The model under review builds one solid part; all positions refer to its coordinate system, in mm. Face numbers are marked on the shaded views. Coordinates: 2 decimals unless noted, no trailing zeros. Write each loop counter-clockwise with the first axis right and the second up, starting at its lowest first coordinate (ties: lowest second). Pieces come first, ordered by that corner, then holes. Notation, with made-up numbers: (-35, 52) - (19, 52) arc R18 cw to (19, 75) - close; hole circle Ø4 at (-39, -7). An arc over 180 degrees is marked (long way). Put each result on its own line as item: value. Start each with the question number.
Item 1: Mouldability with a two-part tool opening along Z and no side actions: class the marked faces 1, 2 and 3 as pulls with the +Z half, pulls with the -Z half, needs draft (parallel to the pull), parting line crosses it, or undercut.
Item 2: Consider section C-C on y = 46.5. State how many separate pieces and enclosed holes the cut face has, then the cut area to 3 significant figures.
Item 3: Consider section B-B on z = 179.75. Give the boundary of the cut face in (x, y), then the cut area to 3 significant figures.
Item 4: To check wall thickness, follow L1, parallel to X at y = 69, z = 134.5; L2, parallel to X at y = 94.5, z = -184.5; L3, parallel to Y at x = -139, z = -8. State the ranges of each line that lie inside material, in increasing order. Write a range as [from, to].
Item 5: For pin 1 (3 mm diameter, centred on x = 152, y = 47.5, fed in from -Z); pin 2 (3 mm diameter, centred on x = 101.5, y = 20.5, fed in from -Z) (3 decimals); pin 3 (4 mm diameter, centred on y = 88, z = -197, fed in from +X), all flat-tipped, find the tip position at first contact; note any pin that passes through.
Item 6: Consider section A-A on x = 0. Give the boundary of the cut face in (y, z), then the cut area to 3 significant figures.
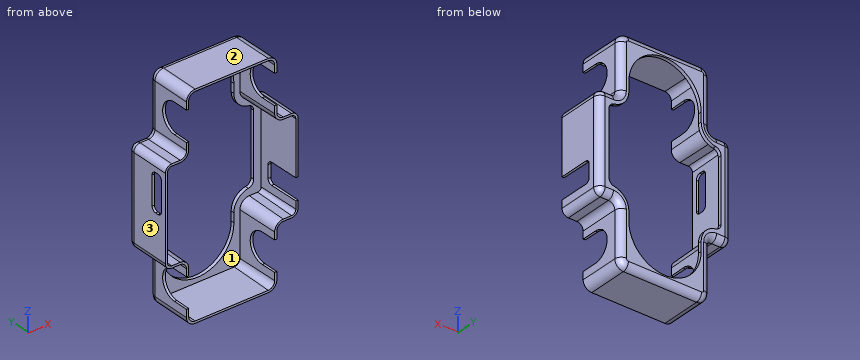
```python
from build123d import *

# Parameters (mm, degrees)
SKETCH1_W           = 310
SKETCH1_H           = 505
BOSS_EXTRUDE1_DEPTH = 108
SKETCH2_W           = 75
SKETCH2_H           = 140
CUT_EXTRUDE1_DEPTH  = 316.349409386
FILLET1_R           = 15
FILLET3_R           = 20
FILLET4_R           = 15
FILLET5_R           = 15
CUT_EXTRUDE2_DEPTH  = 379.524107555
CUT_EXTRUDE3_DEPTH  = 100
CUT_EXTRUDE3_DRAFT  = -1
SKETCH18_W          = 87
SKETCH18_H          = 27.388454903
CUT_EXTRUDE4_DEPTH  = 90
FILLET6_R           = 10
SKETCH19_W          = 50
SKETCH19_H          = 98.394535989
CUT_EXTRUDE5_DEPTH  = 90
FILLET7_R           = 10
CUT_EXTRUDE7_DEPTH  = 90
FILLET12_R          = 40
FILLET13_R          = 15


with BuildPart() as part:
    # Sketch1 → Boss-Extrude1 (new body)
    with BuildSketch(Plane(origin=(0, 0, 0), x_dir=(1, 0, 0), z_dir=(0, 1, 0))):
        Rectangle(SKETCH1_W, SKETCH1_H)
    extrude(amount=BOSS_EXTRUDE1_DEPTH)

    # Sketch2 → Cut-Extrude1 (cut, through all)
    with BuildSketch(Plane(origin=(0, 0, 0), x_dir=(-1, 0, 0), z_dir=(0, -1, 0))):
        with Locations((143, -182.5)):
            Rectangle(SKETCH2_W, SKETCH2_H)
        with Locations((-143, -182.5)):
            Rectangle(SKETCH2_W, SKETCH2_H)
        with Locations((-143, 182.5)):
            Rectangle(SKETCH2_W, SKETCH2_H)
        with Locations((143, 182.5)):
            Rectangle(SKETCH2_W, SKETCH2_H)
    extrude(amount=-CUT_EXTRUDE1_DEPTH, mode=Mode.SUBTRACT)

    # Fillet1
    fillet1_edges = [part.edges().sort_by_distance(p)[0] for p in [
        (-105.5, 54, -112.5),
        (105.5, 54, -112.5),
        (105.5, 54, 112.5),
        (-105.5, 54, 112.5),
    ]]
    fillet(fillet1_edges, radius=FILLET1_R)

    # Fillet3
    fillet3_edges = [part.edges().sort_by_distance(p)[0] for p in [
        (-105.5, 54, -252.5),
        (105.5, 54, -252.5),
        (105.5, 54, 252.5),
        (-105.5, 54, 252.5),
    ]]
    fillet(fillet3_edges, radius=FILLET3_R)

    # Fillet4
    fillet4_edges = [part.edges().sort_by_distance(p)[0] for p in [
        (105.5, 108, 180),
        (0, 108, 252.5),
        (-105.5, 108, -180),
        (0, 108, -252.5),
        (-99.642135624, 108, -246.642135624),
        (99.642135624, 108, -246.642135624),
        (-99.642135624, 108, 246.642135624),
        (99.642135624, 108, 246.642135624),
        (155, 108, 0),
        (-155, 108, 0),
        (137.75, 108, -112.5),
        (-137.75, 108, 112.5),
        (137.75, 108, 112.5),
        (-105.5, 108, 180),
        (105.5, 108, -180),
        (-137.75, 108, -112.5),
        (109.893398282, 108, 116.893398282),
        (-109.893398282, 108, 116.893398282),
        (109.893398282, 108, -116.893398282),
        (-109.893398282, 108, -116.893398282),
    ]]
    fillet(fillet4_edges, radius=FILLET4_R)

    # Fillet5
    # the kernel refuses this fillet: 15 mm, written as the material it takes off along each edge
    with BuildSketch(Plane(origin=(140, 93, -97.5), x_dir=(0, 0, -1), z_dir=(1, 0, 0))) as fillet5_piece_1_section:
        Polygon((0, 0), (FILLET5_R, 0), (FILLET5_R, FILLET5_R), (0, FILLET5_R), align=None)
    fillet5_piece_1 = extrude(amount=FILLET5_R, mode=Mode.PRIVATE)
    fillet5_piece_1 = fillet5_piece_1 - Plane(origin=(140, 93, -97.5), x_dir=(0, -0.7071067811865475, 0.7071067811865475), z_dir=(1, 0, 0)) * Sphere(FILLET5_R, mode=Mode.PRIVATE)
    add(fillet5_piece_1, mode=Mode.SUBTRACT)
    with BuildSketch(Plane(origin=(140, 93, 97.5), x_dir=(1, 0, 0), z_dir=(0, 0, 1))) as fillet5_piece_2_section:
        Polygon((0, 0), (FILLET5_R, 0), (FILLET5_R, FILLET5_R), (0, FILLET5_R), align=None)
    fillet5_piece_2 = extrude(amount=FILLET5_R, mode=Mode.PRIVATE)
    fillet5_piece_2 = fillet5_piece_2 - Plane(origin=(140, 93, 97.5), x_dir=(-0.7071067811865475, -0.7071067811865475, 0), z_dir=(0, 0, 1)) * Sphere(FILLET5_R, mode=Mode.PRIVATE)
    add(fillet5_piece_2, mode=Mode.SUBTRACT)
    with BuildSketch(Plane(origin=(-140, 93, -97.5), x_dir=(0, 0, -1), z_dir=(-1, 0, 0))) as fillet5_piece_3_section:
        Polygon((0, 0), (FILLET5_R, 0), (FILLET5_R, -FILLET5_R), (0, -FILLET5_R), align=None)
    fillet5_piece_3 = extrude(amount=FILLET5_R, mode=Mode.PRIVATE)
    fillet5_piece_3 = fillet5_piece_3 - Plane(origin=(-140, 93, -97.5), x_dir=(0, -0.7071067811865475, 0.7071067811865475), z_dir=(-1, 0, 0)) * Sphere(FILLET5_R, mode=Mode.PRIVATE)
    add(fillet5_piece_3, mode=Mode.SUBTRACT)
    with BuildSketch(Plane(origin=(-140, 93, 97.5), x_dir=(-1, 0, 0), z_dir=(0, 0, 1))) as fillet5_piece_4_section:
        Polygon((0, 0), (FILLET5_R, 0), (FILLET5_R, -FILLET5_R), (0, -FILLET5_R), align=None)
    fillet5_piece_4 = extrude(amount=FILLET5_R, mode=Mode.PRIVATE)
    fillet5_piece_4 = fillet5_piece_4 - Plane(origin=(-140, 93, 97.5), x_dir=(0.7071067811865475, -0.7071067811865475, 0), z_dir=(0, 0, 1)) * Sphere(FILLET5_R, mode=Mode.PRIVATE)
    add(fillet5_piece_4, mode=Mode.SUBTRACT)
    with BuildSketch(Plane(origin=(155, 93, 112.5), x_dir=(-1, 0, 0), z_dir=(0, -1, 0)), Plane(origin=(155, 93, -112.5), x_dir=(0, 0, 1), z_dir=(0, -1, 0))) as fillet5_piece_5:
        with BuildLine():
            CenterArc((FILLET5_R, FILLET5_R), FILLET5_R, 180, 90)
            Line((0, FILLET5_R), (0, 0))
            Line((0, 0), (FILLET5_R, 0))
        make_face()
    extrude(amount=130.5, mode=Mode.SUBTRACT)
    with BuildSketch(Plane(origin=(-155, 93, -112.5), x_dir=(0, 0, 1), z_dir=(0, -1, 0)), Plane(origin=(-155, 93, 112.5), x_dir=(1, 0, 0), z_dir=(0, -1, 0))) as fillet5_piece_6:
        with BuildLine():
            CenterArc((FILLET5_R, -FILLET5_R), FILLET5_R, 90, 90)
            Line((0, -FILLET5_R), (0, 0))
            Line((0, 0), (FILLET5_R, 0))
        make_face()
    extrude(amount=130.5, mode=Mode.SUBTRACT)

    # Sketch16 → Cut-Extrude2 (cut, through all)
    with BuildSketch(Plane.ZY.offset(105.5)):
        with BuildLine():
            Line((-144.75, 35.449402931), (-144.75, -45.449402931))
            ThreePointArc((-144.75, -45.449402931), (-179.75, -80.449402931), (-214.75, -45.449402931))
            Line((-214.75, -45.449402931), (-214.75, 35.449402931))
            ThreePointArc((-214.75, 35.449402931), (-179.75, 70.449402931), (-144.75, 35.449402931))
        make_face()
        with BuildLine():
            Line((144.75, 35.449402931), (144.75, -45.449402931))
            ThreePointArc((144.75, -45.449402931), (179.75, -80.449402931), (214.75, -45.449402931))
            Line((214.75, -45.449402931), (214.75, 35.449402931))
            ThreePointArc((214.75, 35.449402931), (179.75, 70.449402931), (144.75, 35.449402931))
        make_face()
    extrude(amount=-CUT_EXTRUDE2_DEPTH, mode=Mode.SUBTRACT)


with BuildPart() as cut_extrude3_tool:
    # Sketch17 → Cut-Extrude3 (with draft: the straight prism first)
    with BuildSketch(Plane(origin=(0, 0, 0), x_dir=(-1, 0, 0), z_dir=(0, -1, 0))):
        with BuildLine():
            Line((-100.5, -214.75), (-100.5, -232.5))
            ThreePointArc((-100.5, -232.5), (-96.106601718, -243.106601718), (-85.5, -247.5))
            Line((-85.5, -247.5), (85.5, -247.5))
            ThreePointArc((85.5, -247.5), (96.106601718, -243.106601718), (100.5, -232.5))
            Line((100.5, -232.5), (100.5, -214.75))
            Line((100.5, -214.75), (100.5, -144.75))
            Line((100.5, -144.75), (100.5, -127.5))
            ThreePointArc((100.5, -127.5), (106.357864376, -113.357864376), (120.5, -107.5))
            Line((120.5, -107.5), (140, -107.5))
            ThreePointArc((140, -107.5), (147.071067812, -104.571067812), (150, -97.5))
            Line((150, -97.5), (150, 97.5))
            ThreePointArc((150, 97.5), (147.071067812, 104.571067812), (140, 107.5))
            Line((140, 107.5), (120.5, 107.5))
            ThreePointArc((120.5, 107.5), (106.357864376, 113.357864376), (100.5, 127.5))
            Line((100.5, 127.5), (100.5, 144.75))
            Line((100.5, 144.75), (100.5, 214.75))
            Line((100.5, 214.75), (100.5, 232.5))
            ThreePointArc((100.5, 232.5), (96.106601718, 243.106601718), (85.5, 247.5))
            Line((85.5, 247.5), (-85.5, 247.5))
            ThreePointArc((-85.5, 247.5), (-96.106601718, 243.106601718), (-100.5, 232.5))
            Line((-100.5, 232.5), (-100.5, 214.75))
            Line((-100.5, 214.75), (-100.5, 144.75))
            Line((-100.5, 144.75), (-100.5, 127.5))
            ThreePointArc((-100.5, 127.5), (-106.357864376, 113.357864376), (-120.5, 107.5))
            Line((-120.5, 107.5), (-140, 107.5))
            ThreePointArc((-140, 107.5), (-147.071067812, 104.571067812), (-150, 97.5))
            Line((-150, 97.5), (-150, -97.5))
            ThreePointArc((-150, -97.5), (-147.071067812, -104.571067812), (-140, -107.5))
            Line((-140, -107.5), (-120.5, -107.5))
            ThreePointArc((-120.5, -107.5), (-106.357864376, -113.357864376), (-100.5, -127.5))
            Line((-100.5, -127.5), (-100.5, -144.75))
            Line((-100.5, -144.75), (-100.5, -214.75))
        make_face()
    extrude(amount=-CUT_EXTRUDE3_DEPTH)
    # Cut-Extrude3: the draft: its side faces are tilted about the plane it starts from
    cut_extrude3_sides = [cut_extrude3_tool.faces().sort_by_distance(p)[0] for p in [
        (106.357864376, 50, 113.357864376),
        (147.071067812, 50, 104.571067812),
        (150, 50, 0),
        (147.071067812, 50, -104.571067812),
        (130.25, 50, -107.5),
        (106.357864376, 50, -113.357864376),
        (100.5, 50, -180),
        (96.106601718, 50, -243.106601718),
        (0, 50, -247.5),
        (-96.106601718, 50, -243.106601718),
        (-100.5, 50, -180),
        (-106.357864376, 50, -113.357864376),
        (-130.25, 50, -107.5),
        (-147.071067812, 50, -104.571067812),
        (-150, 50, 0),
        (-147.071067812, 50, 104.571067812),
        (-130.25, 50, 107.5),
        (-106.357864376, 50, 113.357864376),
        (-100.5, 50, 180),
        (-96.106601718, 50, 243.106601718),
        (0, 50, 247.5),
        (96.106601718, 50, 243.106601718),
        (100.5, 50, 180),
        (130.25, 50, 107.5),
    ]]
    draft(cut_extrude3_sides, Plane(origin=(0, 0, 0), x_dir=(-1, 0, 0), z_dir=(0, -1, 0)), CUT_EXTRUDE3_DRAFT)


with BuildPart() as part_1:
    add(part.part)

    # Cut-Extrude3: cut by cut_extrude3_tool
    add(cut_extrude3_tool.part, mode=Mode.SUBTRACT)

    # Sketch18 → Cut-Extrude4 (cut)
    with BuildSketch(Plane.ZY.offset(155)):
        with Locations((41.75, 25.394227452)):
            Rectangle(SKETCH18_W, SKETCH18_H)
    extrude(amount=-CUT_EXTRUDE4_DEPTH, mode=Mode.SUBTRACT)

    # Fillet6
    fillet6_edges = [part_1.edges().sort_by_distance(p)[0] for p in [
        (-152.39788787, 11.7, -1.75),
        (-152.158854241, 39.088454903, -1.75),
        (-152.158854241, 39.088454903, 85.25),
        (-152.39788787, 11.7, 85.25),
    ]]
    fillet(fillet6_edges, radius=FILLET6_R)

    # Sketch19 → Cut-Extrude5 (cut)
    with BuildSketch(Plane(origin=(155, 0, 0), x_dir=(0, 0, -1), z_dir=(1, 0, 0))):
        with Locations((54.75, 30.802732005)):
            Rectangle(SKETCH19_W, SKETCH19_H)
    extrude(amount=-CUT_EXTRUDE5_DEPTH, mode=Mode.SUBTRACT)

    # Fillet7
    fillet7_edges = [part_1.edges().sort_by_distance(p)[0] for p in [
        (151.801797403, 80, -29.75),
        (151.801797403, 80, -79.75),
    ]]
    fillet(fillet7_edges, radius=FILLET7_R)

    # Sketch20 → Cut-Extrude7 (cut)
    with BuildSketch(Plane(origin=(0, 108, 0), x_dir=(1, 0, 0), z_dir=(0, 1, 0))):
        with BuildLine():
            Line((-131, -88.5), (-120.5, -88.5))
            ThreePointArc((-120.5, -88.5), (-98.990836138, -94.967618132), (-84.615675262, -112.225340001))
            Line((-84.615675262, -112.225340001), (-84.615675262, -150.25))
            ThreePointArc((-84.615675262, -150.25), (0, -234.865675262), (84.615675262, -150.25))
            Line((84.615675262, -150.25), (84.615675262, -112.225340001))
            ThreePointArc((84.615675262, -112.225340001), (98.990836138, -94.967618132), (120.5, -88.5))
            Line((120.5, -88.5), (131, -88.5))
            Line((131, -88.5), (131, 88.5))
            Line((131, 88.5), (120.5, 88.5))
            ThreePointArc((120.5, 88.5), (98.990836138, 94.967618132), (84.615675262, 112.225340001))
            Line((84.615675262, 112.225340001), (84.615675262, 150.25))
            ThreePointArc((84.615675262, 150.25), (0, 234.865675262), (-84.615675262, 150.25))
            Line((-84.615675262, 150.25), (-84.615675262, 112.225340001))
            ThreePointArc((-84.615675262, 112.225340001), (-98.990836138, 94.967618132), (-120.5, 88.5))
            Line((-120.5, 88.5), (-131, 88.5))
            Line((-131, 88.5), (-131, -88.5))
        make_face()
    extrude(amount=-CUT_EXTRUDE7_DEPTH, mode=Mode.SUBTRACT)

    # Fillet12
    fillet12_edges = [part_1.edges().sort_by_distance(p)[0] for p in [
        (-84.615675262, 104, 112.225340001),
        (84.615675262, 104, 112.225340001),
        (84.615675262, 104, -112.225340001),
        (-84.615675262, 104, -112.225340001),
    ]]
    fillet(fillet12_edges, radius=FILLET12_R)

    # Fillet13
    fillet13_edges = [part_1.edges().sort_by_distance(p)[0] for p in [
        (-131, 104, 88.5),
        (131, 104, -88.5),
        (131, 104, 88.5),
        (-131, 104, -88.5),
    ]]
    fillet(fillet13_edges, radius=FILLET13_R)


solid = part_1.part
```
Report:
1. face 1: undercut
1. face 2: pulls with the +Z half
1. face 3: needs draft
2. separate pieces: 5
2. enclosed holes: 0
2. area: 7,030 mm²
3. outline: (-105.5, 70.45) - (-99.27, 70.45) - (-98.75, 100) - (-79.31, 100) - (-79.31, 108) - (-90.5, 108) arc R15 ccw to (-105.5, 93) - close; (79.31, 100) - (98.75, 100) - (99.27, 70.45) - (105.5, 70.45) - (105.5, 93) arc R15 ccw to (90.5, 108) - (79.31, 108) - close
3. area: 706 mm²
4. L1: [-105.5, -99.3], [99.3, 105.5]
4. L2: [-105.42, -98.85], [98.85, 105.42]
4. L3: [100, 108]
5. pin 1: z = -108.21
5. pin 2: z = -246.275
5. pin 3: x = 105.5
6. outline: (0, -252.5) - (93, -252.5) arc R15 ccw to (108, -237.5) - (108, -234.87) - (100, -234.87) - (100, -245.75) - (0, -247.5) - close; (0, 247.5) - (100, 245.75) - (100, 234.87) - (108, 234.87) - (108, 237.5) arc R15 ccw to (93, 252.5) - (0, 252.5) - close
6. area: 1,360 mm²
